Autodesk Inventor part; units mm, degrees
ref_plane "YZ Plane" through (0, 0, 0) normal (1, 0, 0) x (0, 1, 0)
ref_plane "XZ Plane" through (0, 0, 0) normal (0, 1, 0) x (-1, 0, 0)
ref_plane "XY Plane" through (0, 0, 0) normal (0, 0, 1) x (1, 0, 0)
sketch "Sketch1" plane through (0, 0, 0) normal (0, 0, 1) x (1, 0, 0)
  line L0 (-20, -20) -> (20, -20)
  line L1 (20, -20) -> (20, 20)
  line L2 (20, 20) -> (-20, 20)
  line L3 (-20, 20) -> (-20, -20)
  line L4 (-20, -20) -> (20, 20) construction
  line L5 (20, -20) -> (-20, 20) construction
  point P0 (0, 0)
  dimension "d0" = 40
  dimension "d1" = 40
extrude "Extrusion1" add sketch "Sketch1" along normal blind 5
sketch "Sketch3" plane through (0, 0, 0) normal (0, 0, -1) x (-1, 0, 0)
  line L0 (-20, -20) -> (20, -20)
  line L1 (20, -20) -> (20, 20)
  line L2 (20, 20) -> (-20, 20)
  line L3 (-20, 20) -> (-20, -20)
  line L4 (-20, -20) -> (20, 20) construction
  line L5 (20, -20) -> (-20, 20) construction
  line L6 (-10.1, -10) -> (10.1, -10)
  line L7 (10.1, -10) -> (10.1, 20)
  line L8 (10.1, 20) -> (-10.1, 20)
  line L9 (-10.1, 20) -> (-10.1, -10)
  line L10 (-10.1, -10) -> (10.1, 20) construction
  line L11 (10.1, -10) -> (-10.1, 20) construction
  point P0 (0, 0)
  point P1 (0, 5)
  dimension "d8" = 40
  dimension "d9" = 40
  dimension "d10" = 20.2
  dimension "d11" = 30
  dimension "d55" = 20
extrude "Extrusion3" add sketch "Sketch3" along normal blind 40.1 contours L3 L2 L9 L6 L7 L1 L0
sketch "Sketch4" plane through (0, 0, 0) normal (0, 0, -1) x (-1, 0, 0)
  circle A0 centre (0, 0) radius 7.5
  dimension "d14" = 15
extrude "Extrusion4" cut sketch "Sketch4" against normal blind 6
sketch "Sketch6" plane through (20, -20, -40.1) normal (1, 0, 0) x (0, 0, -1)
  line L0 (-45.1, 40) -> (-37.1, 40)
  line L1 (-37.1, 40) -> (-37.1, 0)
  line L2 (-37.1, 0) -> (-45.1, 0)
  line L3 (-45.1, 0) -> (-45.1, 40)
  line L4 (-45.1, 40) -> (-37.1, 0) construction
  line L5 (-37.1, 40) -> (-45.1, 0) construction
  line L6 (0, 40) -> (-45.1, 40)
  line L7 (-45.1, 0) -> (0, 0)
  line L8 (-45.1, 0) -> (-45.1, 40)
  point P0 (-40.1, 20)
  point P1 (-41.1, 20)
  point P2 (-40.1, 40)
  point P3 (-45.1, 50)
  dimension "d19" = 8
extrude "Extrusion6" add sketch "Sketch6" along normal blind 15
mirror "Mirror1" about plane through (0, 0, 0) normal (1, 0, 0) of "Extrusion6"
sketch "Sketch7" plane through (0, 0, 5) normal (0, 0, 1) x (1, 0, 0)
  circle A0 centre (27.5, 10) radius 2.05
  circle A1 centre (27.5, -10) radius 2.05
  circle A2 centre (-27.5, -10) radius 2.05
  circle A3 centre (-27.5, 10) radius 2.05
  line L0 (35, 20) -> (35, -20)
  line L1 (-35, 20) -> (-35, -20)
  line L2 (35, -20) -> (-35, -20)
  line L3 (-35, 20) -> (35, 20)
  line L4 (-20, 20) -> (-35, 20)
  point P0 (0, 0)
  point P1 (20, 20)
  dimension "d22" = 4.1
  dimension "d23" = 4.1
  dimension "d24" = 4.1
  dimension "d25" = 4.1
  dimension "d26" = 7.5
  dimension "d27" = 7.5
  dimension "d28" = 7.5
  dimension "d29" = 7.5
  dimension "d30" = 10
  dimension "d31" = 10
  dimension "d32" = 10
  dimension "d33" = 10
extrude "Extrusion7" cut sketch "Sketch7" against normal blind 45.1 contours A0 | A1 | A2 | A3
sketch "Sketch9" plane through (20, -20, -3) normal (0, 0, -1) x (-1, 0, 0)
  circle A0 centre (-7.5, 30) radius 2.05
  circle A1 centre (-7.5, 10) radius 2.05
  circle A2 centre (47.5, 30) radius 2.05
  circle A3 centre (47.5, 10) radius 2.05
  circle A4 centre (-7.5, 30) radius 5
  circle A5 centre (-7.5, 10) radius 5
  circle A6 centre (47.5, 30) radius 5
  circle A7 centre (47.5, 10) radius 5
  point P0 (20, 20)
  dimension "d39" = 10
  dimension "d40" = 10
  dimension "d41" = 10
  dimension "d42" = 10
extrude "Extrusion8" cut sketch "Sketch9" against normal blind 5 contours A0 | A1 | A4 | A5 | A6 | A7
sketch "Sketch10" plane through (-20, -20, -40.1) normal (-1, 0, 0) x (0, 0, 1)
  line L0 (22.1, 17.5) -> (37.1, 17.5)
  line L1 (37.1, 17.5) -> (37.1, 32.5)
  line L2 (37.1, 32.5) -> (22.1, 32.5)
  line L3 (22.1, 32.5) -> (22.1, 17.5)
  line L4 (22.1, 17.5) -> (37.1, 32.5) construction
  line L5 (37.1, 17.5) -> (22.1, 32.5) construction
  line L6 (37.1, 0) -> (37.1, 40)
  line L7 (40.1, 10) -> (0, 10)
  point P0 (40.1, 20)
  point P1 (29.6, 25)
  dimension "d45" = 15
  dimension "d46" = 15
  dimension "d47" = 7.5
extrude "Extrusion9" cut sketch "Sketch10" against normal through all
sketch "Sketch11" plane through (-20, -20, -40.1) normal (0, -1, 0) x (1, 0, 0)
  line L0 (27.5, 22.1) -> (12.5, 22.1)
  line L1 (12.5, 22.1) -> (12.5, 37.1)
  line L2 (12.5, 37.1) -> (27.5, 37.1)
  line L3 (27.5, 37.1) -> (27.5, 22.1)
  line L4 (27.5, 22.1) -> (12.5, 37.1) construction
  line L5 (12.5, 22.1) -> (27.5, 37.1) construction
  line L6 (0, 37.1) -> (-15, 37.1)
  line L7 (0, 0) -> (0, 37.1)
  point P0 (20, 40.1)
  point P1 (20, 29.6)
  dimension "d50" = 15
  dimension "d51" = 15
  dimension "d52" = 20
extrude "Extrusion10" cut sketch "Sketch11" against normal through all
sketch "Sketch12" plane through (0, 0, 0) normal (0, 0, -1) x (-1, 0, 0)
  ellipse E0 centre (7.952, -7.882) end of major axis (8.818, -8.748) minor radius 1 (8.1756, -9) -> (9.07, -8.1056) ccw
  line L0 (-8.1756, -9) -> (8.1756, -9)
  ellipse E1 centre (-7.952, -7.882) end of major axis (-8.818, -8.748) minor radius 1 (-9.07, -8.1056) -> (-8.1756, -9) ccw
  line L1 (-9.07, 28.2056) -> (-9.07, -8.1056)
  ellipse E2 centre (-7.952, 27.982) end of major axis (-8.818, 28.848) minor radius 1 (-8.1756, 29.1) -> (-9.07, 28.2056) ccw
  line L2 (8.1756, 29.1) -> (-8.1756, 29.1)
  ellipse E3 centre (7.952, 27.982) end of major axis (8.818, 28.848) minor radius 1 (9.07, 28.2056) -> (8.1756, 29.1) ccw
  line L3 (9.07, -8.1056) -> (9.07, 28.2056)
  circle A0 centre (-7.525, 27.6) radius 0.7835
  circle A1 centre (7.525, 27.6) radius 0.7835
  circle A2 centre (-7.525, 12.5) radius 0.7835
  circle A3 centre (7.525, 12.5) radius 0.7835
  circle A4 centre (-7.525, -7.5) radius 0.7835
  circle A5 centre (7.525, -7.5) radius 0.7835
  circle A6 centre (0, 0) radius 6.4
  point P0 (0, 0)
hole "Hole1" at (-7.525, -7.5, 0) at (-7.525, 12.5, 0) at (7.525, 12.5, 0) at (7.525, -7.5, 0) direction (0, 0, 1) diameter 2.1 end through all
sketch "Sketch13" plane through (0, 0, 5) normal (0, 0, 1) x (1, 0, 0)
  circle A0 centre (-7.525, 12.5) radius 1.05
  circle A1 centre (7.525, 12.5) radius 1.05
  circle A2 centre (-7.525, 12.5) radius 2
  circle A3 centre (7.525, 12.5) radius 2
  point P0 (0, 0)
  dimension "d63" = 4
  dimension "d64" = 4
extrude "Extrusion11" cut sketch "Sketch13" against normal blind 2.5 contours A0 | A1 | A2 | A3
mirror "Mirror2" about plane through (0, 0, 0) normal (1, 0, 0)
sketch "Sketch16" plane through (0, 0, -40.1) normal (0, 0, -1) x (-1, 0, 0)
  circle A0 centre (37.5, 12.5) radius 2.05
  line L0 (45, -20) -> (45, 20)
  line L1 (10.1, 20) -> (45, 20)
  circle A1 centre (37.5, -12.5) radius 2.05
  circle A2 centre (-37.5, 12.5) radius 2.05
  circle A3 centre (-37.5, -12.5) radius 2.05
  line L2 (45, -20) -> (-45, -20)
  line L3 (-45, -20) -> (-45, 20)
  line L4 (-10.1, 20) -> (-20, 20)
  point P0 (0, 0)
  dimension "d74" = 4.1
  dimension "d75" = 7.5
  dimension "d76" = 7.5
  dimension "d77" = 4.1
  dimension "d78" = 4.1
  dimension "d79" = 4.1
  dimension "d80" = 7.5
  dimension "d81" = 7.5
  dimension "d82" = 7.5
  dimension "d83" = 7.5
  dimension "d84" = 7.5
  dimension "d85" = 7.5
extrude "Extrusion14" cut sketch "Sketch16" against normal through all
sketch "Sketch18" plane through (0, 0, 5) normal (0, 0, 1) x (1, 0, 0)
  circle A0 centre (7.525, -7.5) radius 1.05
  circle A1 centre (-7.525, -7.5) radius 1.05
  circle A2 centre (7.525, -7.5) radius 2
  circle A3 centre (-7.525, -7.5) radius 2
  point P0 (0, 0)
  dimension "d94" = 4
  dimension "d95" = 4
extrude "Extrusion16" cut sketch "Sketch18" against normal blind 2.5
sketch "Sketch19" plane through (0, 0, -40.1) normal (0, 0, -1) x (-1, 0, 0)
  line L0 (20, 20) -> (20, -20)
  line L1 (20, -20) -> (35, -20)
  line L2 (35, -20) -> (35, 20)
  line L3 (-35, -20) -> (-20, -20)
  line L4 (-20, -20) -> (-20, 20)
  line L5 (-20, 20) -> (-35, 20)
  line L6 (-35, 20) -> (-35, -20)
  line L7 (-35, -20) -> (-20, 20) construction
  line L8 (-20, -20) -> (-35, 20) construction
  line L9 (20, 20) -> (35, 20)
  line L10 (20, -20) -> (20, 20)
  line L11 (20, 20) -> (35, 20)
  line L12 (35, -20) -> (35, 20)
  line L13 (20, -20) -> (35, -20)
  line L14 (-20, 20) -> (-20, -20)
  line L15 (-20, 20) -> (-35, 20)
  line L16 (-35, -20) -> (-35, 20)
  line L17 (-20, -20) -> (-35, -20)
  point P0 (0, 0)
  point P1 (-27.5, 0)
extrude "Extrusion17" add sketch "Sketch19" against normal blind 5
sketch "Sketch20" plane through (0, 0, -40.1) normal (0, 0, -1) x (-1, 0, 0)
  circle A0 centre (-27.5, 10) radius 2.05
  circle A1 centre (-27.5, -10) radius 2.05
  circle A2 centre (27.5, -10) radius 2.05
  circle A3 centre (27.5, 10) radius 2.05
  circle A4 centre (-27.5, 10) radius 2.05
  circle A5 centre (-27.5, -10) radius 2.05
  circle A6 centre (27.5, 10) radius 2.05
  circle A7 centre (27.5, -10) radius 2.05
  point P0 (0, 0)
extrude "Extrusion18" cut sketch "Sketch20" against normal blind 10
ref_plane "Work Plane1" through (0, 0, 0) normal (1, 0, 0) x (0, 1, 0)
properties part number "motor1_bracket" material "ABS Plastic"
Work out the finished part from the listing and answer in its coordinate system (mm). A direction names the side the tool comes from. Round coordinates to 2 decimals unless told otherwise and drop trailing zeros. Write each loop counter-clockwise with the first axis right and the second up, starting at its lowest first coordinate (ties: lowest second). Pieces come first, ordered by that corner, then holes. Notation, with made-up numbers: M 48.25,41 L 84.25,41 A28 ccw 84.25,74 Z; hole C 62.5,82 d1. An arc over 180 degrees is marked long. Use a Markdown table: item, result.
1) Determine the mould class of faces 4 (the face through (29.55, -9.91, -37.64)), 5 (the face through (-22.505, 10.22, -0.535)), 6 (the face through (8.4, -8.4, 2.5)) for opening direction Z: pulls with the +Z half, pulls with the -Z half, needs draft (parallel to the pull), parting line crosses it, or undercut.
Taken from the geometry:
| item | result |
|---|---|
| face 4 | needs draft |
| face 5 | undercut |
| face 6 | pulls with the +Z half |
2) Consider line 1 (X direction, y = 10, z = 3); line 2 (Y direction, x = -27.5, z = 0.95); line 3 (X direction, y = 11, z = -25). Determine where each line is inside the solid, lowest interval first. Write a range as [from, to].
Taken from the geometry:
| item | result |
|---|---|
| line 1 | x = [-35, -29.55], [-25.45, 25.45], [29.55, 35] |
| line 2 | y = [-20, -15], [-5, 5], [15, 20] |
| line 3 | x = [-20, -10.1], [10.1, 20] |
3) Which of the six approach directions +Z, -Z, +X, -X, +Y, -Y give full straight-line access (tool end or side, diameter ignored) to faces 1 (the face through (32.495, -9.78, -0.535)), 2 (the face through (-7.5, -15, -11)), 3 (the face through (8.4, 11.6, 2.5))?
Taken from the geometry:
| item | result |
|---|---|
| face 1 | none |
| face 2 | +Y, -Y |
| face 3 | +Z |
4) The part is cut by section D-D on x = 0. Give the vertices of the cut face in (y, z), plus the area to 3 significant figures.
Taken from the geometry:
| item | result |
|---|---|
| outline | M -20,-40.1 L -10,-40.1 L -10,-18 L -20,-18 Z; M -20,-3 L -10,-3 L -10,0 L -7.5,0 L -7.5,5 L -20,5 Z; M 7.5,0 L 20,0 L 20,5 L 7.5,5 Z |
| area | 376 mm2 |
5) The part is cut by section C-C on x = -27.5. State how many separate pieces and enclosed holes the cut face has, plus the area to 3 significant figures.
Taken from the geometry:
| item | result |
|---|---|
| separate pieces | 6 |
| enclosed holes | 0 |
| area | 354 mm2 |
6) The part is cut by section B-B on z = -2. Give the vertices of the cut face in (x, y).
Taken from the geometry:
| item | result |
|---|---|
| outline | M -35,-20 L 35,-20 L 35,20 L 10.1,20 L 10.1,-10 L -10.1,-10 L -10.1,20 L -35,20 Z; hole C -27.5,-10 d10; hole C -27.5,10 d10; hole C 27.5,-10 d10; hole C 27.5,10 d10 |
7) The part is cut by section A-A on y = 0. Give the vertices of the cut face in (x, z), plus the area to 3 significant figures.
Taken from the geometry:
| item | result |
|---|---|
| outline | M -35,-40.1 L -10.1,-40.1 L -10.1,-18 L -20,-18 L -20,-35.1 L -35,-35.1 Z; M -35,-3 L -10.1,-3 L -10.1,0 L -7.5,0 L -7.5,5 L -35,5 Z; M 7.5,0 L 10.1,0 L 10.1,-3 L 35,-3 L 35,5 L 7.5,5 Z; M 10.1,-40.1 L 35,-40.1 L 35,-35.1 L 20,-35.1 L 20,-18 L 10.1,-18 Z |
| area | 1,010 mm2 |
8) Flat-ended cylindrical pins translate along their axes: pin 1 (2.5 mm diameter, centred on x = 7.525, y = 12.5, fed in from +Z); pin 2 (2.5 mm diameter, centred on x = 7.525, y = -7.5, fed in from -Z); pin 3 (1.5 mm diameter, centred on y = 3, z = -23, fed in from -X). Find the tip coordinate at first contact, or state that the pin passes through.
Taken from the geometry:
| item | result |
|---|---|
| pin 1 | stops at z = 2.5 |
| pin 2 | stops at z = 0 |
| pin 3 | stops at x = -20 |
